The listing builds one solid part. Answer for the finished solid, in the listing's coordinates (mm). Coordinates: 2 decimals unless noted, no trailing zeros. Answer as CSV lines item,"result". Start each with the question number.
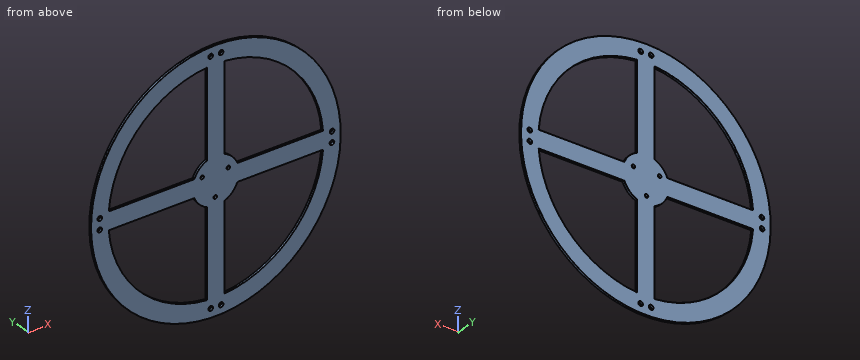
```python
from build123d import *

# Parameters (mm, degrees)
SKETCH1_R           = 107.5
SKETCH1_R_2         = 2
BOSS_EXTRUDE1_DEPTH = 2
SKETCH2_R           = 1.5
CUT_EXTRUDE1_DEPTH  = 153.041112861
FILLET1_R           = 0.1


with BuildPart() as part:
    # Sketch1 → Boss-Extrude1 (new body)
    with BuildSketch(Plane(origin=(0, 0, 0), x_dir=(1, 0, 0), z_dir=(0, 1, 0))):
        with Locations(Location((0, 0, 0), (0, 0, 270))):
            Circle(SKETCH1_R)
        with Locations(Location((-4.5, -100, 0), (0, 0, 270))):
            Circle(SKETCH1_R_2, mode=Mode.SUBTRACT)
        with Locations(Location((-99.89869869, -4.5, 0), (0, 0, 270))):
            Circle(SKETCH1_R_2, mode=Mode.SUBTRACT)
        with BuildLine():
            ThreePointArc((-7.5, -92.195444573), (-65.40737726, -65.40737726), (-92.195444573, -7.5))
            Line((-92.195444573, -7.5), (-18.540496218, -7.5))
            ThreePointArc((-18.540496218, -7.5), (-14.142135624, -14.142135624), (-7.5, -18.540496218))
            Line((-7.5, -18.540496218), (-7.5, -92.195444573))
        make_face(mode=Mode.SUBTRACT)
        with Locations(Location((4.5, -99.89869869, 0), (0, 0, 270))):
            Circle(SKETCH1_R_2, mode=Mode.SUBTRACT)
        with BuildLine():
            Line((7.5, -92.195444573), (7.5, -18.540496218))
            ThreePointArc((7.5, -18.540496218), (14.142135624, -14.142135624), (18.540496218, -7.5))
            Line((18.540496218, -7.5), (92.195444573, -7.5))
            ThreePointArc((92.195444573, -7.5), (65.40737726, -65.40737726), (7.5, -92.195444573))
        make_face(mode=Mode.SUBTRACT)
        with Locations(Location((100, -4.5, 0), (0, 0, 270))):
            Circle(SKETCH1_R_2, mode=Mode.SUBTRACT)
        with Locations(Location((-100, 4.5, 0), (0, 0, 270))):
            Circle(SKETCH1_R_2, mode=Mode.SUBTRACT)
        with BuildLine():
            ThreePointArc((-92.195444573, 7.5), (-65.40737726, 65.40737726), (-7.5, 92.195444573))
            Line((-7.5, 92.195444573), (-7.5, 18.540496218))
            ThreePointArc((-7.5, 18.540496218), (-14.142135624, 14.142135624), (-18.540496218, 7.5))
            Line((-18.540496218, 7.5), (-92.195444573, 7.5))
        make_face(mode=Mode.SUBTRACT)
        with Locations(Location((-4.5, 99.89869869, 0), (0, 0, 270))):
            Circle(SKETCH1_R_2, mode=Mode.SUBTRACT)
        with BuildLine():
            Line((7.5, 18.540496218), (7.5, 92.195444573))
            ThreePointArc((7.5, 92.195444573), (65.40737726, 65.40737726), (92.195444573, 7.5))
            Line((92.195444573, 7.5), (18.540496218, 7.5))
            ThreePointArc((18.540496218, 7.5), (14.142135624, 14.142135624), (7.5, 18.540496218))
        make_face(mode=Mode.SUBTRACT)
        with Locations(Location((99.89869869, 4.5, 0), (0, 0, 270))):
            Circle(SKETCH1_R_2, mode=Mode.SUBTRACT)
        with Locations(Location((4.5, 100, 0), (0, 0, 270))):
            Circle(SKETCH1_R_2, mode=Mode.SUBTRACT)
    extrude(amount=BOSS_EXTRUDE1_DEPTH)

    # Sketch2 → Cut-Extrude1 (cut, through all)
    with BuildSketch(Plane.XZ):
        with Locations(Location((-11.820616269, 6.611877399, 0), (0, 0, 270))):
            Circle(SKETCH2_R)
        with Locations(Location((-0.56228602, -12.888122601, 0), (0, 0, 270))):
            Circle(SKETCH2_R)
        with Locations(Location((10.696044229, 6.611877399, 0), (0, 0, 270))):
            Circle(SKETCH2_R)
    extrude(amount=-CUT_EXTRUDE1_DEPTH, mode=Mode.SUBTRACT)

    # Fillet1
    fillet1_edges = [part.edges().sort_by_distance(p)[0] for p in [
        (7.5, 2, 55.367970395),
        (14.142135624, 2, 14.142135624),
        (55.367970395, 2, 7.5),
        (0, 2, -107.5),
        (-65.40737726, 2, -65.40737726),
        (-7.5, 2, -55.367970395),
        (-14.142135624, 2, -14.142135624),
        (0, 0, -107.5),
        (-55.367970395, 2, -7.5),
        (7.5, 2, -55.367970395),
        (65.40737726, 2, -65.40737726),
        (55.367970395, 2, -7.5),
        (14.142135624, 2, -14.142135624),
        (-65.40737726, 2, 65.40737726),
        (-55.367970395, 2, 7.5),
        (-14.142135624, 2, 14.142135624),
        (-7.5, 2, 55.367970395),
        (65.40737726, 2, 65.40737726),
    ]]
    fillet(fillet1_edges, radius=FILLET1_R)


solid = part.part
```
Item 1: Consider line 1 (X direction, y = 0.8, z = 4.5); line 2 (X direction, y = 1, z = -4.5); line 3 (Z direction, x = -15.5, y = 0.4). Determine where each line is inside the solid, lowest interval first.
Item 2: Each of these flat-tipped pins is pushed along its axis until it touches: P1, Ø3, axis at x = 4.5, z = 99.9, coming from the -Y side; P2, Ø1, axis at x = -68, y = 1, coming from the +Z side; P3, Ø1, axis at y = 1, z = -63.5, coming from the +X side. Where does it stop, or does it pass through?
Item 3: Section A-A on y = 1.2 is taken. State how many separate pieces and enclosed holes the cut face has, then the cut area to 3 significant figures.
Results are:
1,line 1,"-107.41 to -101.9, -97.9 to 98, 102 to 107.41"
1,line 2,"-107.41 to -102, -98 to 97.9, 101.9 to 107.41"
1,line 3,"-106.38 to -91.19, -12.64 to 12.64, 91.19 to 106.38"
2,P1,"through"
2,P2,"z = 83.67"
2,P3,"x = 87.1"
3,separate pieces,"1"
3,enclosed holes,"15"
3,area,"14,900 mm²"
